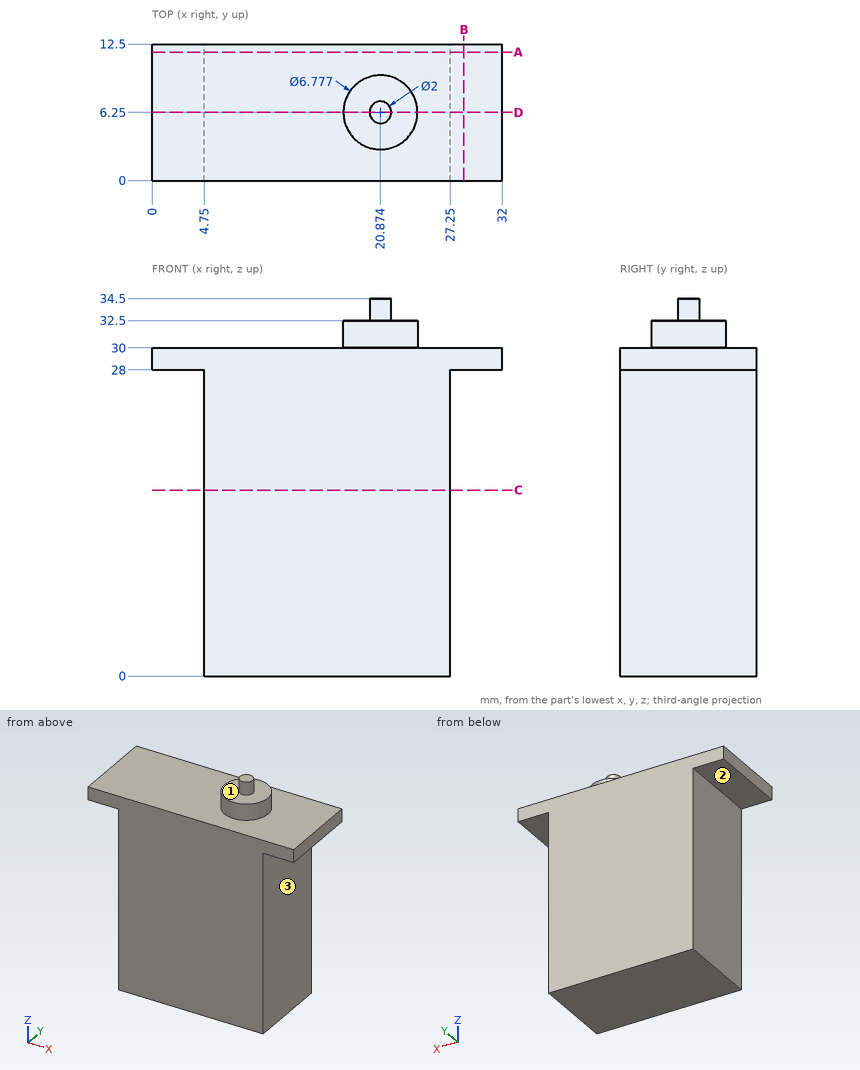
Could you check a few things on this drawing? It's one solid part, dimensions in mm from its lowest x, y, z. A direction names the side the tool comes from. Round coordinates to 2 decimals unless told otherwise and drop trailing zeros. Loops run counter-clockwise (first coordinate to the right, second up) from the corner with the lowest first, then second, coordinate; pieces in that order, holes last. Notation, with made-up numbers: (89, 79) -> (144, 79) arc R24 cw to (144, 102) -> close; hole circle Ø4 at (-23, 48). An arc over 180 degrees is marked (long way). One line per item, written item: value. Start each with the question number.
1. If we section it at C-C, the plane z = 17: Write out the boundary of the cut face in (x, y).
2. If we section it at A-A, the plane y = 11.75: Write out the boundary of the cut face in (x, z), then the cut area to 3 significant figures.
3. If we section it at D-D, the plane y = 6.25: Write out the boundary of the cut face in (x, z).
4. If I drill on probe 1 along X at (y, z) = (11.25, 25); probe 2 along Z at (x, y) = (4.5, 7.75); probe 3 along Z at (x, y) = (17, 10), over which ranges is the centre line in solid material (lowest first)?
5. If we section it at B-B, the plane x = 28.5: Write out the boundary of the cut face in (y, z), then the cut area to 3 significant figures.
6. For the marked faces 1, 2 and 3, which set-ups out of +Z, -Z, +X, -X, +Y, -Y let a thin tool reach every point of the face, with its end or its side?
7. For pin 1 (6 mm diameter, centred on y = 5, z = 17.5, fed in from -X); pin 2 (1.4 mm diameter, centred on x = 29.5, y = 8, fed in from -Z); pin 3 (6 mm diameter, centred on x = 13.5, y = 7.5, fed in from +Z), each with a flat end and sliding along its axis, tell me the tip position at first contact or that it passes through.
Calculated:
1. outline: (4.75, 0) -> (27.25, 0) -> (27.25, 12.5) -> (4.75, 12.5) -> close
2. outline: (0, 28) -> (4.75, 28) -> (4.75, 0) -> (27.25, 0) -> (27.25, 28) -> (32, 28) -> (32, 30) -> (0, 30) -> close
2. area: 694 mm²
3. outline: (0, 28) -> (4.75, 28) -> (4.75, 0) -> (27.25, 0) -> (27.25, 28) -> (32, 28) -> (32, 30) -> (24.26, 30) -> (24.26, 32.5) -> (21.87, 32.5) -> (21.87, 34.5) -> (19.87, 34.5) -> (19.87, 32.5) -> (17.49, 32.5) -> (17.49, 30) -> (0, 30) -> close
4. probe 1: x = 4.75 to 27.25
4. probe 2: z = 28 to 30
4. probe 3: z = 0 to 30
5. outline: (0, 28) -> (12.5, 28) -> (12.5, 30) -> (0, 30) -> close
5. area: 25.0 mm²
6. face 1: +Z
6. face 2: -Z, -X, +Y, -Y
6. face 3: -Z, +X, +Y, -Y
7. pin 1: stops at x = 4.75
7. pin 2: stops at z = 28
7. pin 3: stops at z = 30
